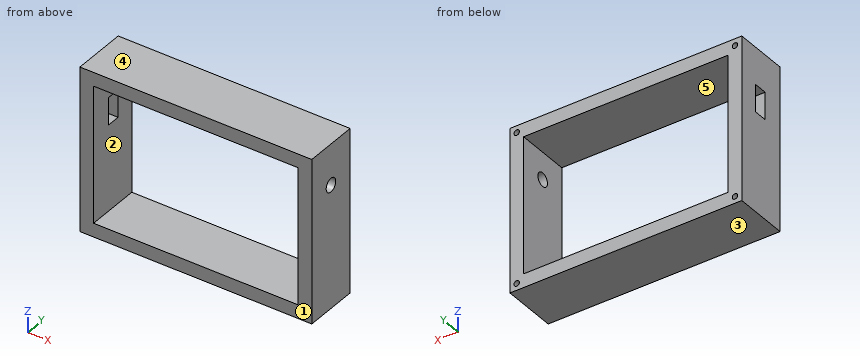
```python
from build123d import *

# Parameters (mm, degrees)
SKETCH1_W                 = 170
SKETCH1_H                 = 120
SKETCH1_W_2               = 150
SKETCH1_H_2               = 100
EXTRUDE_THIN1_DEPTH       = 40
SKETCH2_R                 = 5
CUT_EXTRUDE1_DEPTH        = 10
F_4_0MM_DOWEL_HOLE1_D     = 4
F_4_0MM_DOWEL_HOLE1_DEPTH = 5
F_4_0MM_DOWEL_HOLE1_TIP   = 1.201721238
F_4_0MM_DOWEL_HOLE2_D     = 4
F_4_0MM_DOWEL_HOLE2_DEPTH = 5
F_4_0MM_DOWEL_HOLE2_TIP   = 1.201721238
F_4_0MM_DOWEL_HOLE3_D     = 4
F_4_0MM_DOWEL_HOLE3_DEPTH = 5
F_4_0MM_DOWEL_HOLE3_TIP   = 1.201721238
F_4_0MM_DOWEL_HOLE4_D     = 4
F_4_0MM_DOWEL_HOLE4_DEPTH = 5
F_4_0MM_DOWEL_HOLE4_TIP   = 1.201721238
SKETCH15_W                = 20
SKETCH15_H                = 10
CUT_EXTRUDE7_DEPTH        = 10


with BuildPart() as part:
    # Sketch1 → Extrude-Thin1 (new body)
    with BuildSketch(Plane(origin=(0, 0, 0), x_dir=(1, 0, 0), z_dir=(0, 1, 0))):
        Rectangle(SKETCH1_W, SKETCH1_H)
        Rectangle(SKETCH1_W_2, SKETCH1_H_2, mode=Mode.SUBTRACT)
    extrude(amount=EXTRUDE_THIN1_DEPTH)

    # Sketch2 → Cut-Extrude1 (cut)
    with BuildSketch(Plane(origin=(85, 0, 0), x_dir=(0, 0, -1), z_dir=(1, 0, 0))):
        with Locations((-30, 20)):
            Circle(SKETCH2_R)
    extrude(amount=-CUT_EXTRUDE1_DEPTH, mode=Mode.SUBTRACT)

    # Ø4.0mm Dowel Hole1
    with Locations(Plane(origin=(0, 40, 0), x_dir=(1, 0, 0), z_dir=(0, 1, 0))):
        with Locations((-80, 55)):
            Hole(F_4_0MM_DOWEL_HOLE1_D / 2, depth=F_4_0MM_DOWEL_HOLE1_DEPTH)
            with Locations((0, 0, -(F_4_0MM_DOWEL_HOLE1_DEPTH + F_4_0MM_DOWEL_HOLE1_TIP / 2))):  # 118° drill point
                Cone(0, F_4_0MM_DOWEL_HOLE1_D / 2, F_4_0MM_DOWEL_HOLE1_TIP, mode=Mode.SUBTRACT)

    # Ø4.0mm Dowel Hole2
    with Locations(Plane(origin=(0, 40, 0), x_dir=(1, 0, 0), z_dir=(0, 1, 0))):
        with Locations((-80, -55)):
            Hole(F_4_0MM_DOWEL_HOLE2_D / 2, depth=F_4_0MM_DOWEL_HOLE2_DEPTH)
            with Locations((0, 0, -(F_4_0MM_DOWEL_HOLE2_DEPTH + F_4_0MM_DOWEL_HOLE2_TIP / 2))):  # 118° drill point
                Cone(0, F_4_0MM_DOWEL_HOLE2_D / 2, F_4_0MM_DOWEL_HOLE2_TIP, mode=Mode.SUBTRACT)

    # Ø4.0mm Dowel Hole3
    with Locations(Plane(origin=(0, 40, 0), x_dir=(1, 0, 0), z_dir=(0, 1, 0))):
        with Locations((80, -55)):
            Hole(F_4_0MM_DOWEL_HOLE3_D / 2, depth=F_4_0MM_DOWEL_HOLE3_DEPTH)
            with Locations((0, 0, -(F_4_0MM_DOWEL_HOLE3_DEPTH + F_4_0MM_DOWEL_HOLE3_TIP / 2))):  # 118° drill point
                Cone(0, F_4_0MM_DOWEL_HOLE3_D / 2, F_4_0MM_DOWEL_HOLE3_TIP, mode=Mode.SUBTRACT)

    # Ø4.0mm Dowel Hole4
    with Locations(Plane(origin=(0, 40, 0), x_dir=(1, 0, 0), z_dir=(0, 1, 0))):
        with Locations((80, 55)):
            Hole(F_4_0MM_DOWEL_HOLE4_D / 2, depth=F_4_0MM_DOWEL_HOLE4_DEPTH)
            with Locations((0, 0, -(F_4_0MM_DOWEL_HOLE4_DEPTH + F_4_0MM_DOWEL_HOLE4_TIP / 2))):  # 118° drill point
                Cone(0, F_4_0MM_DOWEL_HOLE4_D / 2, F_4_0MM_DOWEL_HOLE4_TIP, mode=Mode.SUBTRACT)

    # Sketch15 → Cut-Extrude7 (cut)
    with BuildSketch(Plane.ZY.offset(85)):
        with Locations((22.785330455, 20.631239888)):
            Rectangle(SKETCH15_W, SKETCH15_H)
    extrude(amount=-CUT_EXTRUDE7_DEPTH, mode=Mode.SUBTRACT)


solid = part.part
```
Verification items for the finished model (mm, model axes). Face numbers are marked on the shaded views. A direction names the side the tool comes from. Round coordinates to 2 decimals unless told otherwise and drop trailing zeros. Write each loop counter-clockwise with the first axis right and the second up, starting at its lowest first coordinate (ties: lowest second). Pieces come first, ordered by that corner, then holes. Notation, with made-up numbers: (33.5, -28.5) - (66.5, -28.5) arc R37 ccw to (66.5, 10.5) - close; hole circle Ø6 at (24, -34). An arc over 180 degrees is marked (long way). Answer as a JSON object with one key per item and string values. Group by question number.
Q1. Go/stop test with flat-tipped pins: pin 1 Ø13 at (y, z) = (20, 30) entering from -X; pin 2 Ø2.5 at (x, z) = (-80, -55) entering from +Y. Record where each tip stops, or that it passes through.
Q2. Section check C-C, the plane x = 28. Enter the section's corners in (y, z).
Q3. Mould release check, pull along Z, two halves, no side actions. Record for the marked faces 3, 4 and 5: released by +Z, released by -Z, zero draft, split by the parting line, or undercut.
Q4. Tool access check on the marked faces 1 and 2. Record the directions out of +Z, -Z, +X, -X, +Y, -Y that give a thin tool (end or side, any length) a straight path to the whole face; none if there is none.
Q5. Thickness scan on line 1 (X direction, y = 37, z = 55); line 2 (Z direction, x = -80, y = 38.95); line 3 (Z direction, x = -19, y = 12.5). Record the ranges inside material, lowest first.
Q6. Section check D-D, the plane y = 8. Enter the section's corners in (x, z).
Q7. Section check B-B, the plane z = 30. Enter the section's corners in (x, y), plus the area to 3 significant figures.
Q8. Section check A-A, the plane z = 9.5. Enter the section's corners in (x, y), plus the area to 3 significant figures.
Found:
{
 "1": {"pin 1": "stops at x = -85", "pin 2": "stops at y = 34.55"},
 "2": {"outline": "(0, -60) - (40, -60) - (40, -50) - (0, -50) - close; (0, 50) - (40, 50) - (40, 60) - (0, 60) - close"},
 "3": {"face 3": "released by -Z", "face 4": "released by +Z", "face 5": "undercut"},
 "4": {"face 1": "+Z, -Z, +X, -X, -Y", "face 2": "+Y, -Y"},
 "5": {"line 1": "x = -85 to -82, -78 to 78, 82 to 85", "line 2": "z = -60 to -57, -53 to 53, 57 to 60", "line 3": "z = -60 to -50, 50 to 60"},
 "6": {"outline": "(-85, -60) - (85, -60) - (85, 60) - (-85, 60) - close; hole (-75, -50) - (75, -50) - (75, 50) - (-75, 50) - close"},
 "7": {"outline": "(-85, 0) - (-75, 0) - (-75, 15.63) - (-85, 15.63) - close; (-85, 25.63) - (-75, 25.63) - (-75, 40) - (-85, 40) - close; (75, 0) - (85, 0) - (85, 15) - (75, 15) - close; (75, 25) - (85, 25) - (85, 40) - (75, 40) - close", "area": "600 mm^2"},
 "8": {"outline": "(-85, 0) - (-75, 0) - (-75, 40) - (-85, 40) - close; (75, 0) - (85, 0) - (85, 40) - (75, 40) - close", "area": "800 mm^2"}
}
